Part print with two shaded views. Sizes in mm from the minimum x, y, z corner. A direction names the side the tool comes from. Round coordinates to 2 decimals unless told otherwise and drop trailing zeros. Loops run counter-clockwise (first coordinate to the right, second up) from the corner with the lowest first, then second, coordinate; pieces in that order, holes last. Notation, with made-up numbers: M -37.5,6.5 L 13.5,6.5 A26 ccw 13.5,28.5 Z; hole C 36,59.5 d1. An arc over 180 degrees is marked long. Put each result on its own line as item: value. Start each with the question number.
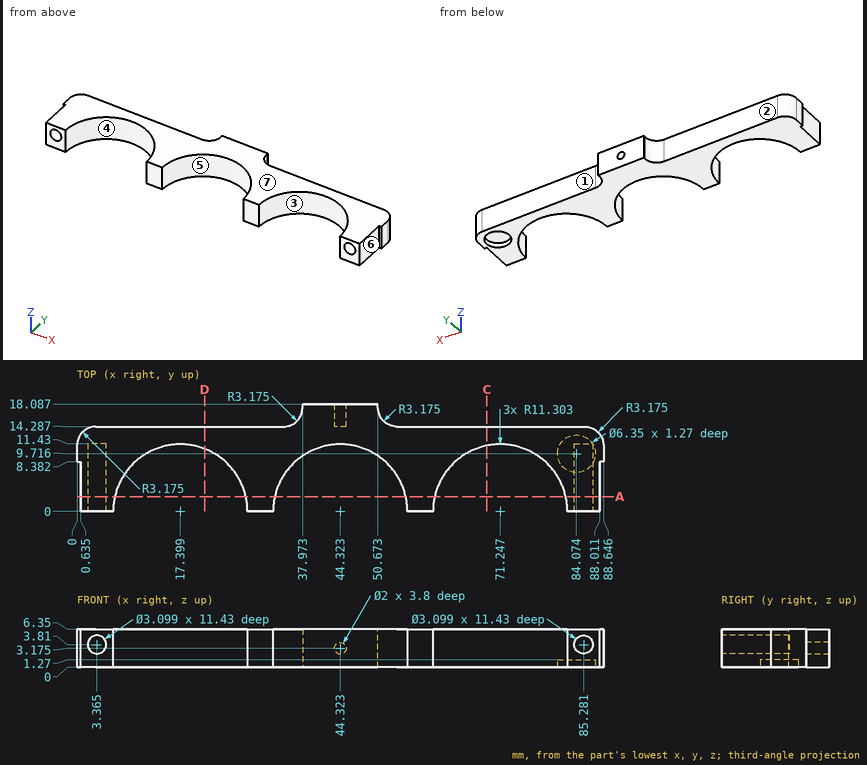
(1) Tool access for the marked faces 1, 2 and 3: list every direction of +Z, -Z, +X, -X, +Y, -Y with a clear straight run to the whole face (end or side of a thin tool).
(2) Cut at D-D on x = 21.5. List the corners of the cut face in (y, z).
(3) Drill centre lines: line 1 along Z through (x, y) = (44.5, 15.25); line 2 along Y through (x, z) = (56, 6.25); line 3 along Y through (x, z) = (46, 3.5). Where is each one in solid material? Low to high.
(4) Cut at A-A on y = 2.5. Count the separate pieces of the cut face and the enclosed holes in it, and give its area (3 significant figures).
(5) Mould opens along X. For the marked faces 4, 5, 6 and 7 say: +X half, -X half, draft (parallel to the pull), parting line (faces both ways), or undercut.
(6) Flat gauge pins, fed straight in: pin 1 Ø1.2 at (x, z) = (44.323, 3.175) entering from -Y; pin 2 Ø1.9 at (x, z) = (26, 2) entering from +Y; pin 3 Ø3 at (x, y) = (82.5, 9.5) entering from -Z. Where does each tip first touch, or does it go through?
(7) Cut at C-C on x = 69. List the corners of the cut face in (y, z).
Taken from the geometry:
1. face 1: +Z, -Z, +X, +Y
1. face 2: +Z, -Z, -X, +Y
1. face 3: +Z, -Z, -Y
2. outline: M 10.53,0 L 14.29,0 L 14.29,6.35 L 10.53,6.35 Z
3. line 1: 0 to 2.19, 4.16 to 6.35
3. line 2: 0 to 14.29
3. line 3: 11.18 to 18.09
4. separate pieces: 4
4. enclosed holes: 2
4. area: 120 mm2
5. face 4: undercut
5. face 5: undercut
5. face 6: +X half
5. face 7: draft
6. pin 1: y = 11.29
6. pin 2: y = 14.29
6. pin 3: z = 1.27
7. outline: M 11.08,0 L 14.29,0 L 14.29,6.35 L 11.08,6.35 Z
